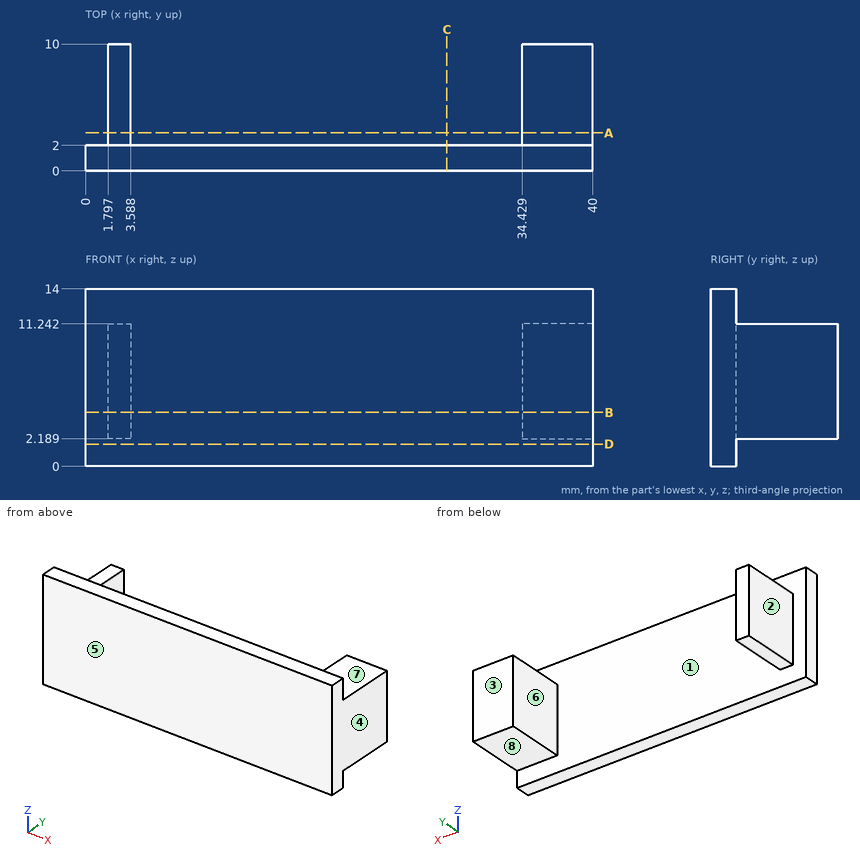
Print and shaded views of the part. All mm, measured from the part's lowest x, y and z. A direction names the side the tool comes from. Round coordinates to 2 decimals unless told otherwise and drop trailing zeros. Write each loop counter-clockwise with the first axis right and the second up, starting at its lowest first coordinate (ties: lowest second). Pieces come first, ordered by that corner, then holes.
(1) Slice it at C-C, the plane x = 28.5. Write the cut outline in (y, z), and give its area (3 significant figures).
(2) Slice it at D-D, the plane z = 1.75. Write the cut outline in (x, y).
(3) Probe line 1 along X through (y, z) = (7.75, 4.5); line 2 along Y through (x, z) = (26, 12); line 3 along Z through (x, y) = (34.5, 2.25). List the from-to ranges inside material, lowest first.
(4) Slice it at B-B, the plane z = 4.25. Write the cut outline in (x, y).
(5) Slice it at A-A, the plane y = 3. Write the cut outline in (x, z).
(6) Mould opens along X. For the marked faces 1, 2, 3 and 4 say: pulls with the +X half, pulls with the -X half, needs draft (parallel to the pull), parting line crosses it, or undercut.
(7) Drop flat-ended pins along their axis: P1, Ø2, axis at x = 2.5, y = 4.5, coming from the -Z side; P2, Ø4, axis at x = 33, z = 10.5, coming from the -Y side; P3, Ø0.9, axis at x = 3, y = 6, coming from the +Z side; P4, Ø2, axis at y = 7, z = 5, coming from the -X side. Give the stop position or say it passes through.
(8) 3-axis set-ups, long thin cutter, end or side, ignore diameter. For the marked faces 5, 6, 7 and 8: which of +Z, -Z, +X, -X, +Y, -Y reach the whole face in a straight line?
From the geometry:
1. outline: (0, 0) - (2, 0) - (2, 14) - (0, 14) - close
1. area: 28.0 mm2
2. outline: (0, 0) - (40, 0) - (40, 2) - (0, 2) - close
3. line 1: x = 1.8 to 3.59, 34.43 to 40
3. line 2: y = 0 to 2
3. line 3: z = 2.19 to 11.24
4. outline: (0, 0) - (40, 0) - (40, 10) - (34.43, 10) - (34.43, 2) - (3.59, 2) - (3.59, 10) - (1.8, 10) - (1.8, 2) - (0, 2) - close
5. outline: (1.8, 2.19) - (3.59, 2.19) - (3.59, 11.24) - (1.8, 11.24) - close; (34.43, 2.19) - (40, 2.19) - (40, 11.24) - (34.43, 11.24) - close
6. face 1: undercut
6. face 2: pulls with the -X half
6. face 3: needs draft
6. face 4: pulls with the +X half
7. P1: stops at z = 2.19
7. P2: stops at y = 0
7. P3: stops at z = 11.24
7. P4: stops at x = 1.8
8. face 5: +Z, -Z, +X, -X, -Y
8. face 6: +Z, -Z, +Y
8. face 7: +Z, +X, -X, +Y
8. face 8: -Z, +X, -X, +Y
